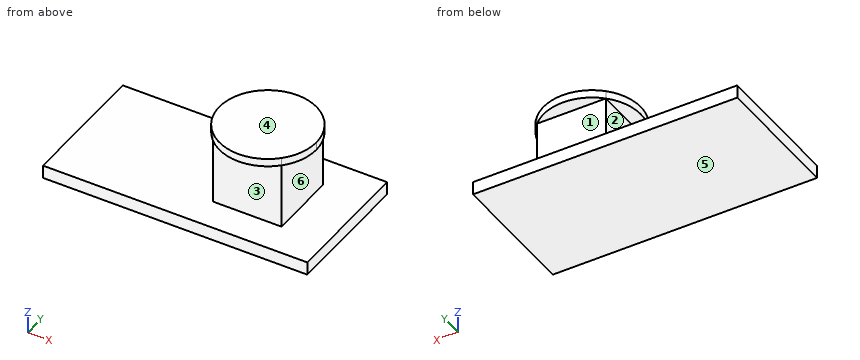
```python
from build123d import *

# Parameters (mm, degrees)
F0_W     = 20
F0_H     = 12
F0_H_2   = 20
F0_W_2   = 17
F0_H_3   = 3
F0_W_3   = 3
F0_W_4   = 10.8891367149
F0_H_4   = 26
F1_DEPTH = 5
F2_DEPTH = 30
F4_DEPTH = 3


# Not quite as in the source:
# - a feature names something its author has since deleted; it is built from what else it names


with BuildPart() as f1:
    # F0 (on Top) → F1 (new body)
    with BuildSketch(Plane.XY):
        Polygon((-50, 25), (-50, -25), (-3.8891367149, -25), (-3.8891367149, -13), (-3.8891367149, 13), (-3.8891367149, 25), align=None)
        Polygon((-3.8891367149, -13), (-3.8891367149, -25), (10, -25), (10, -13), (7, -13), align=None)
        with Locations((20, -19)):
            Rectangle(F0_W, F0_H)
        Polygon((30, -13), (30, -25), (50, -25), (50, -13), (33, -13), align=None)
        Polygon((50, 25), (30, 25), (30, 13), (33, 13), (50, 13), align=None)
        with Locations((20, 0)):
            Rectangle(F0_W, F0_H_2)
        with Locations((41.5, 0)):
            Rectangle(F0_W_2, F0_H_2)
        with Locations((20, 19)):
            Rectangle(F0_W, F0_H)
        with Locations((20, 11.5)):
            Rectangle(F0_W, F0_H_3)
        with Locations((31.5, 11.5)):
            Rectangle(F0_W_3, F0_H_3)
        with Locations((41.5, 11.5)):
            Rectangle(F0_W_2, F0_H_3)
        with Locations((31.5, 0)):
            Rectangle(F0_W_3, F0_H_2)
        with Locations((41.5, -11.5)):
            Rectangle(F0_W_2, F0_H_3)
        with Locations((31.5, -11.5)):
            Rectangle(F0_W_3, F0_H_3)
        with Locations((20, -11.5)):
            Rectangle(F0_W, F0_H_3)
        with Locations((1.5554316426, 0)):
            Rectangle(F0_W_4, F0_H_4)
        Polygon((10, 25), (-3.8891367149, 25), (-3.8891367149, 13), (7, 13), (10, 13), align=None)
        Polygon((7, -13), (10, -13), (10, -10), (10, 10), (10, 13), (7, 13), align=None)
    extrude(amount=F1_DEPTH)

    # F0 (on Top) → F2 (join)
    with BuildSketch(Plane.XY):
        with Locations((20, 11.5)):
            Rectangle(F0_W, F0_H_3)
        with Locations((31.5, 11.5)):
            Rectangle(F0_W_3, F0_H_3)
        with Locations((31.5, 0)):
            Rectangle(F0_W_3, F0_H_2)
        with Locations((31.5, -11.5)):
            Rectangle(F0_W_3, F0_H_3)
        with Locations((20, -11.5)):
            Rectangle(F0_W, F0_H_3)
        Polygon((7, -13), (10, -13), (10, -10), (10, 10), (10, 13), (7, 13), align=None)
    extrude(amount=F2_DEPTH)

    # F3 (on face) → F4 (join)
    with BuildSketch(Plane.XY.offset(30)):
        with BuildLine():
            ThreePointArc((38.3847763109, 0), (36.9853185434, 7.0355493019), (33, 13))
            Line((33, 13), (20, 0))
            Line((20, 0), (33, -13))
            ThreePointArc((33, -13), (36.9853185434, -7.0355493019), (38.3847763109, 0))
        make_face()
        with BuildLine():
            Line((20, 0), (33, 13))
            ThreePointArc((33, 13), (20, 18.3847763109), (7, 13))
            Line((7, 13), (20, 0))
        make_face()
        with BuildLine():
            Line((33, -13), (20, 0))
            Line((20, 0), (7, -13))
            ThreePointArc((7, -13), (20, -18.3847763109), (33, -13))
        make_face()
        Polygon((7, -13), (20, 0), (7, 13), align=None)
        with BuildLine():
            Line((7, -13), (7, 13))
            ThreePointArc((7, 13), (1.6152236891, 0), (7, -13))
        make_face()
    extrude(amount=F4_DEPTH)


solid = f1.part
```
Verification items for the finished model (mm, model axes). Face numbers are marked on the shaded views. A direction names the side the tool comes from. Give positions to 0.01 mm unless a question says otherwise; leave off trailing zeros. Order: outer loops, then holes, each group sorted by start corner. A loop starts at its lowest first (then second) coordinate and runs counter-clockwise, first axis right, second up. Notation, with made-up numbers: (0.25, -38) -> (26.25, -38) arc R29 ccw to (26.25, -15) -> close; hole circle Ø9 at (-40, 4.5). An arc over 180 degrees is marked (long way). One line per item, written item: value.
(1) Draft check along Z on the marked faces 4, 5 and 6. Enter one of: pulls with the +Z half, pulls with the -Z half, needs draft (parallel to the pull), parting line crosses it, or undercut.
Final values:
face 4: pulls with the +Z half
face 5: pulls with the -Z half
face 6: undercut
(2) Sectioned sample at C-C on z = 17. Record the cut outline in (x, y).
Final values:
outline: (7, -13) -> (33, -13) -> (33, 13) -> (7, 13) -> close; hole (10, -10) -> (30, -10) -> (30, 10) -> (10, 10) -> close
(3) Sectioned sample at D-D on y = 5. Record the cut outline in (x, z).
Final values:
outline: (-50, 0) -> (50, 0) -> (50, 5) -> (33, 5) -> (33, 30) -> (37.69, 30) -> (37.69, 33) -> (2.31, 33) -> (2.31, 30) -> (7, 30) -> (7, 5) -> (-50, 5) -> close; hole (10, 5) -> (30, 5) -> (30, 30) -> (10, 30) -> close
(4) Gauge pin test, flat ends, axial feed: pin 1 (1.5 mm diameter, centred on y = 2, z = 28, fed in from +X); pin 2 (3 mm diameter, centred on x = -18, y = 11.5, fed in from +Z); pin 3 (6 mm diameter, centred on x = 17, z = 18.5, fed in from -Y). Record the tip position at first contact, or that the pin passes through.
Final values:
pin 1: x = 33
pin 2: z = 5
pin 3: y = -13
(5) Sectioned sample at B-B on x = 13. Record the cut outline in (y, z).
Final values:
outline: (-25, 0) -> (25, 0) -> (25, 5) -> (13, 5) -> (13, 30) -> (17, 30) -> (17, 33) -> (-17, 33) -> (-17, 30) -> (-13, 30) -> (-13, 5) -> (-25, 5) -> close; hole (-10, 5) -> (10, 5) -> (10, 30) -> (-10, 30) -> close
(6) Scan lines: line 1 along Y through (x, z) = (24.5, 24.5); line 2 along X through (y, z) = (-0.5, 6.5); line 3 along Z through (x, y) = (24.5, 8). Record each from-to range of solid material in increasing order. Write a range as [from, to].
Final values:
line 1: [-13, -10], [10, 13]
line 2: [7, 10], [30, 33]
line 3: [0, 5], [30, 33]
(7) Sectioned sample at A-A on y = -17. Record the cut outline in (x, z).
Final values:
outline: (-50, 0) -> (50, 0) -> (50, 5) -> (-50, 5) -> close; (13, 30) -> (27, 30) -> (27, 33) -> (13, 33) -> close
(8) Tool access check on the marked faces 1, 2 and 3. Record the directions out of +Z, -Z, +X, -X, +Y, -Y that give a thin tool (end or side, any length) a straight path to the whole face; none if there is none.
Final values:
face 1: +X, -X, +Y
face 2: -X, +Y, -Y
face 3: +X, -X, -Y
